For this review, take the finished solid that the model builds, in its own axes (mm). A direction names the side the tool comes from. Coordinates: 2 decimals unless noted, no trailing zeros. Loops run counter-clockwise (first coordinate to the right, second up) from the corner with the lowest first, then second, coordinate; pieces in that order, holes last. Notation, with made-up numbers: (27.5, 27.25) - (37.5, 27.25) arc R11 cw to (37.5, 35.25) - close; hole circle Ø9 at (33.25, 78). An arc over 180 degrees is marked (long way). Answer as a JSON object with one key per item and string values. Group by question number.
Item 1: To check wall thickness, follow line 1 (X direction, y = -9.5, z = 2); line 2 (Y direction, x = -29, z = 19.75); line 3 (Z direction, x = -7, y = -32). State the ranges of each line that lie inside material, in increasing order.
Item 2: We need section B-B (z = 6.5). Give the boundary of the cut face in (x, y).
Item 3: We need section C-C (x = -26). Give the boundary of the cut face in (y, z).
Item 4: Mouldability with a two-part tool opening along Y and no side actions: class faces 4 (the cylindrical face through (-43.196, -68.289, 13.804)), 5 (the flat face through (-41, -64, 15)), 6 (the flat face through (29, -68, 16)) as released by +Y, released by -Y, zero draft, split by the parting line, or undercut.
Item 5: Tool access review of faces 1 (the flat face through (-17.6, -68, 9)), 2 (the flat face through (-1, -66, 18)), 3 (the flat face through (43, -60, 15)): name each direction out of +Z, -Z, +X, -X, +Y, -Y from which nothing blocks a thin tool from reaching the whole face with its end or side.
Item 6: Clearance check with flat-ended pins moving along their axes: pin 1 (2 mm diameter, centred on x = 43, z = 16.5, fed in from -Y); pin 2 (1.2 mm diameter, centred on y = 67.5, z = 10, fed in from -X); pin 3 (10 mm diameter, centred on x = -5.5, y = 8, fed in from +Z). State where each tip first meets the part, or that it passes through.
Item 7: We need section D-D (y = 12). Give the boundary of the cut face in (x, z), then the cut area to 3 significant figures.
from build123d import *

# Parameters (mm, degrees)
SKETCH1_W           = 140
SKETCH1_H           = 90
BOSS_EXTRUDE1_DEPTH = 3
SKETCH2_W           = 4
SKETCH2_H           = 4
SKETCH2_W_2         = 35.2
BOSS_EXTRUDE2_DEPTH = 25
SKETCH4_W           = 55.5
SKETCH4_H           = 40.7
CUT_EXTRUDE1_DEPTH  = 1.5
SKETCH5_W           = 90.034346747
SKETCH5_H           = 4
SKETCH5_W_2         = 90.027377931
BOSS_EXTRUDE3_DEPTH = 12
SKETCH8_W           = 4
SKETCH8_H           = 10
BOSS_EXTRUDE5_DEPTH = 25
FILLET1_START       = -1
FILLET1_DEPTH       = 29


with BuildPart() as part:
    # Sketch1 → Boss-Extrude1 (new body)
    with BuildSketch(Plane(origin=(0, 0, 0), x_dir=(0, 1, 0), z_dir=(0, 0, 1))):
        Rectangle(SKETCH1_W, SKETCH1_H)
    extrude(amount=BOSS_EXTRUDE1_DEPTH)

    # Sketch2 → Boss-Extrude2 (add)
    with BuildSketch(Plane.XY.offset(3)):
        with Locations((-43, 68)):
            Rectangle(SKETCH2_W, SKETCH2_H)
        with Locations((43, 68)):
            Rectangle(SKETCH2_W, SKETCH2_H)
        with Locations((43, -68)):
            Rectangle(SKETCH2_W, SKETCH2_H)
        with Locations((-43, -68)):
            Rectangle(SKETCH2_W, SKETCH2_H)
        with Locations((0, 68)):
            Rectangle(SKETCH2_W_2, SKETCH2_H)
        with Locations((0, -68)):
            Rectangle(SKETCH2_W_2, SKETCH2_H)
    extrude(amount=BOSS_EXTRUDE2_DEPTH)

    # Sketch4 → Cut-Extrude1 (cut)
    with BuildSketch(Plane.XY.offset(3)):
        Rectangle(SKETCH4_W, SKETCH4_H)
    extrude(amount=-CUT_EXTRUDE1_DEPTH, mode=Mode.SUBTRACT)

    # Sketch5 → Boss-Extrude3 (add)
    with BuildSketch(Plane.XY.offset(28)):
        with Locations((0.017173374, -68)):
            Rectangle(SKETCH5_W, SKETCH5_H)
        with Locations((0.013688966, 68)):
            Rectangle(SKETCH5_W_2, SKETCH5_H)
    extrude(amount=-BOSS_EXTRUDE3_DEPTH)

    # Sketch8 → Boss-Extrude5 (add, through all)
    with BuildSketch(Plane.XY.offset(3)):
        with Locations((-43, 65)):
            Rectangle(SKETCH8_W, SKETCH8_H)
        with Locations((43, 65)):
            Rectangle(SKETCH8_W, SKETCH8_H)
        with Locations((43, -65)):
            Rectangle(SKETCH8_W, SKETCH8_H)
        with Locations((-43, -65)):
            Rectangle(SKETCH8_W, SKETCH8_H)
    extrude(amount=BOSS_EXTRUDE5_DEPTH)

    # Fillet1: read off the stored shape, not the designer's step
    # Fillet1 outline → Fillet1 (cut)
    with BuildSketch(Plane.XY.offset(FILLET1_START)):
        with BuildLine():
            Line((45.027377931, 66), (45.027377931, 70))
            Line((45.027377931, 70), (39.370523681, 70))
            ThreePointArc((39.370523681, 70), (42.834625296, 68.898979486), (45.027377931, 66))
        make_face()
        with BuildLine():
            Line((45.034346747, -70), (45.034346747, -66))
            ThreePointArc((45.034346747, -66), (42.841594113, -68.898979486), (39.377492498, -70))
            Line((39.377492498, -70), (45.034346747, -70))
        make_face()
        with BuildLine():
            Line((-39, 70), (-45, 70))
            Line((-45, 70), (-45, 64))
            ThreePointArc((-45, 64), (-43.242640687, 68.242640687), (-39, 70))
        make_face()
        with BuildLine():
            ThreePointArc((-39, -70), (-43.242640687, -68.242640687), (-45, -64))
            Line((-45, -64), (-45, -70))
            Line((-45, -70), (-39, -70))
        make_face()
    extrude(amount=FILLET1_DEPTH, mode=Mode.SUBTRACT)


solid = part.part
Check sheet entries:
{
 "1": {"line 1": "x = -45 to -27.75, 27.75 to 45", "line 2": "y = -70 to -66, 66 to 70", "line 3": "z = 0 to 3"},
 "2": {"outline": "(-45, -64) arc R6 ccw to (-41, -69.66) - (-41, -60) - (-45, -60) - close; (-45, 60) - (-41, 60) - (-41, 69.66) arc R6 ccw to (-45, 64) - close; (-17.6, -70) - (17.6, -70) - (17.6, -66) - (-17.6, -66) - close; (-17.6, 66) - (17.6, 66) - (17.6, 70) - (-17.6, 70) - close; (41, -69.78) arc R6 ccw to (45, -66.09) - (45, -60) - (41, -60) - close; (41, 60) - (45, 60) - (45, 66.08) arc R6 ccw to (41, 69.77) - close"},
 "3": {"outline": "(-70, 0) - (70, 0) - (70, 3) - (20.35, 3) - (20.35, 1.5) - (-20.35, 1.5) - (-20.35, 3) - (-70, 3) - close; (-70, 16) - (-66, 16) - (-66, 28) - (-70, 28) - close; (66, 16) - (70, 16) - (70, 28) - (66, 28) - close"},
 "4": {"face 4": "released by -Y", "face 5": "undercut", "face 6": "zero draft"},
 "5": {"face 1": "+Y, -Y", "face 2": "+Z", "face 3": "+Z, +X, -X"},
 "6": {"pin 1": "stops at y = -69.4", "pin 2": "stops at x = -44.25", "pin 3": "stops at z = 1.5"},
 "7": {"outline": "(-45, 0) - (45, 0) - (45, 3) - (27.75, 3) - (27.75, 1.5) - (-27.75, 1.5) - (-27.75, 3) - (-45, 3) - close", "area": "187 mm2"}
}
